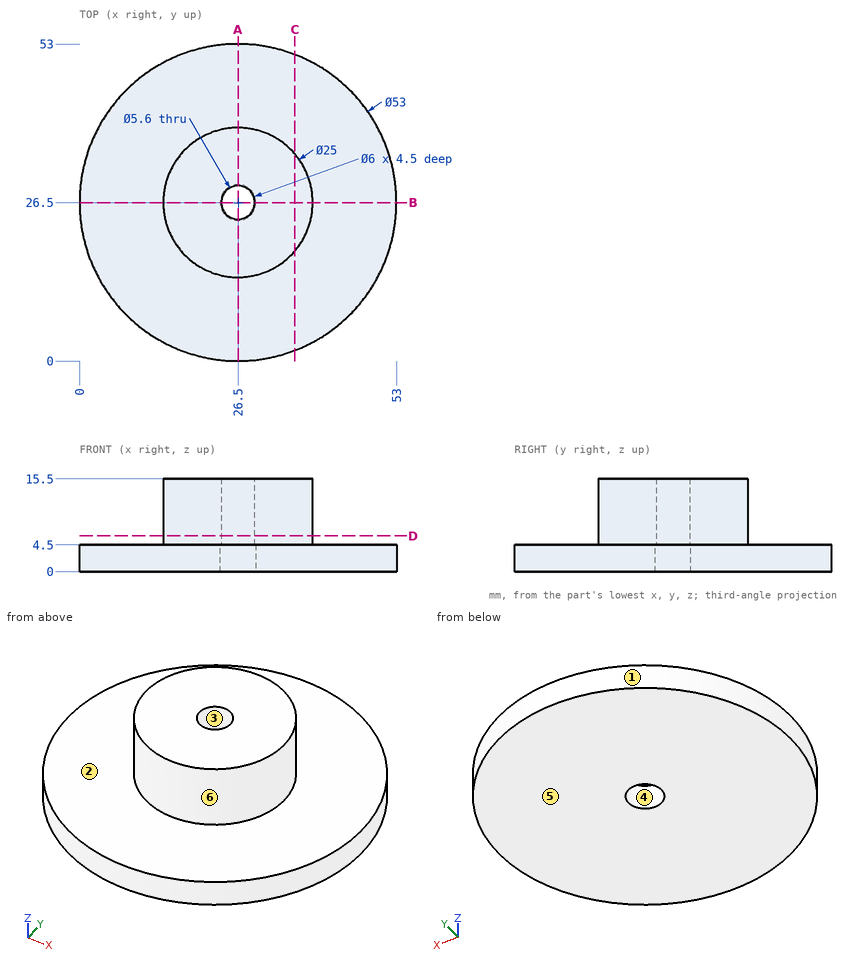
Answer from the drawing. Dimensions are ordinates in mm from the lowest x, y and z of the part. A direction names the side the tool comes from. Give positions to 0.01 mm unless a question says otherwise; leave off trailing zeros. Loops run counter-clockwise (first coordinate to the right, second up) from the corner with the lowest first, then second, coordinate; pieces in that order, holes last. Notation, with made-up numbers: (51.5, -32.75) - (81.5, -32.75) arc R26 ccw to (81.5, -7.75) - close; hole circle Ø5 at (63, 55.25). An arc over 180 degrees is marked (long way). Answer as a JSON object with one key per item and string values.
1. A cutting plane is placed at C-C (x = 36). Write down the section's boundary in (y, z), then the cut area to 3 significant figures.
Determined:
{"outline": "(1.76, 0) - (51.24, 0) - (51.24, 4.5) - (34.62, 4.5) - (34.62, 15.5) - (18.38, 15.5) - (18.38, 4.5) - (1.76, 4.5) - close", "area": "401 mm²"}
2. A cutting plane is placed at A-A (x = 26.5). Write down the section's boundary in (y, z).
Determined:
{"outline": "(0, 0) - (23.5, 0) - (23.5, 4.5) - (23.7, 4.5) - (23.7, 15.5) - (14, 15.5) - (14, 4.5) - (0, 4.5) - close; (29.3, 4.5) - (29.5, 4.5) - (29.5, 0) - (53, 0) - (53, 4.5) - (39, 4.5) - (39, 15.5) - (29.3, 15.5) - close"}
3. For a pull along X with two mould halves and no side action, classify the marked faces 1, 2 and 3 as pulls with the +X half, pulls with the -X half, needs draft (parallel to the pull), parting line crosses it, or undercut.
Determined:
{"face 1": "parting line crosses it", "face 2": "needs draft", "face 3": "undercut"}
4. For the marked faces 4, 5 and 6, determine the directions among +Z, -Z, +X, -X, +Y, -Y from which every point of the face is accessible in a straight line to the end or side of a thin tool.
Determined:
{"face 4": "-Z", "face 5": "-Z, +X, -X, +Y, -Y", "face 6": "+Z"}
5. A cutting plane is placed at D-D (z = 6). Write down the section's boundary in (x, y), then the cut area to 3 significant figures.
Determined:
{"outline": "circle Ø25 at (26.5, 26.5); hole circle Ø5.6 at (26.5, 26.5)", "area": "466 mm²"}
6. Find the intervals of material crossed by L1, parallel to Y at x = 26.5, z = 3.3; L2, parallel to Y at x = 26.5, z = 7; L3, parallel to Z at x = 47, y = 27, in increasing order. Write a range as [from, to].
Determined:
{"L1": "[0, 23.5], [29.5, 53]", "L2": "[14, 23.7], [29.3, 39]", "L3": "[0, 4.5]"}
7. Flat-ended cylindrical pins translate along their axes: pin 1 Ø10 at (x, y) = (19, 35) entering from -Z; pin 2 Ø5 at (x, z) = (13, 10) entering from +Y; pin 3 Ø1.5 at (x, z) = (16.5, 10) entering from +Y; pin 4 Ø6 at (x, z) = (25.5, 3) entering from +Y. Find the tip coordinate at first contact, or state that the pin passes through.
Determined:
{"pin 1": "z = 0", "pin 2": "y = 32.44", "pin 3": "y = 34.91", "pin 4": "y = 53"}
